Here's how the part is built. I have some questions about the finished solid (model axes, mm). Face numbers are marked on the shaded views. A direction names the side the tool comes from. Give positions to 0.01 mm unless a question says otherwise; leave off trailing zeros. Loops run counter-clockwise (first coordinate to the right, second up) from the corner with the lowest first, then second, coordinate; pieces in that order, holes last. Notation, with made-up numbers: (33.25, 76) -> (55.25, 76) arc R33 ccw to (55.25, 106) -> close; hole circle Ø4 at (-1.5, 32.5). An arc over 180 degrees is marked (long way). Answer in a Markdown table with one row per item. Add a question column.
Item 1: We'd pull the mould along Z, two halves only. Please class the marked faces 1, 2, 3 and 4: released by +Z, released by -Z, zero draft, split by the parting line, or undercut.
Item 2: If I drill on line 1 (Y direction, x = 21, z = 0); line 2 (Y direction, x = -7, z = 0); line 3 (Z direction, x = -8, y = 46), over which ranges is the centre line in solid material (lowest first)?
Item 3: If we section it at C-C (z = 0): Give the number of separate pieces and of enclosed holes in the cut face, then the cut area to 3 significant figures.
Item 4: Which directions (+Z, -Z, +X, -X, +Y, -Y) give clear straight access to the entire face, cutting with the end or side of a thin tool? Please do the marked faces 5, 6 and 7.
Item 5: If we section it at B-B (y = 4): Write out the boundary of the cut face in (x, z), then the cut area to 3 significant figures.
Item 6: For P1, Ø12, axis at x = 18.5, y = 21, coming from the +Z side (1 decimal); P2, Ø6, axis at x = 10, y = 47.5, coming from the +Z side; P3, Ø2.5, axis at x = -8.5, z = 1.5, coming from the -Y side; P4, Ø2, axis at x = 12, y = 8, coming from the -Z side, each with a flat end and sliding along its axis, tell me the tip position at first contact or that it passes through.
Item 7: If we section it at A-A (x = 0): Write out the boundary of the cut face in (y, z).
Item 8: If we section it at D-D (x = 13): Write out the boundary of the cut face in (y, z).
Autodesk Inventor part; units mm, degrees
ref_plane "YZ Plane" through (0, 0, 0) normal (1, 0, 0) x (0, 1, 0)
ref_plane "XZ Plane" through (0, 0, 0) normal (0, 1, 0) x (-1, 0, 0)
ref_plane "XY Plane" through (0, 0, 0) normal (0, 0, 1) x (1, 0, 0)
sketch "Sketch1" plane through (0, 0, 0) normal (0, 1, 0) x (-1, 0, 0)
  circle A0 centre (0, 0) radius 6.15
  line L0 (10, 13) -> (-10, 13)
  line L1 (-10, 13) -> (-10, -13)
  line L2 (-10, -13) -> (10, -13)
  line L3 (10, -13) -> (10, 13)
  dimension "d0" = 12.3
  dimension "d1" = 10
  dimension "d2" = 10
  dimension "d3" = 13
  dimension "d4" = 13
extrude "Extrusion1" add sketch "Sketch1" along normal blind 55
sketch "Sketch2" plane through (10, 0, 13) normal (1, 0, 0) x (0, 0, -1)
  circle A0 centre (13, 4) radius 1.45
  line L0 (0, 0) -> (26, 0)
  circle A1 centre (13, 46) radius 1.45
  line L1 (0, 0) -> (0, 55)
  point P0 (13, 0)
  dimension "d7" = 2.9
  dimension "d8" = 4
  dimension "d9" = 2.9
  dimension "d10" = 46
  dimension "d11" = 13
  dimension "d12" = 13
extrude "Extrusion2" cut sketch "Sketch2" against normal blind 55
sketch "Sketch3" plane through (10, 0, 13) normal (1, 0, 0) x (0, 0, -1)
  circle A0 centre (13, 4) radius 1.45
  circle A1 centre (13, 46) radius 1.45
  line L0 (0, 0) -> (26, 0)
  line L1 (26, 0) -> (26, 55)
  line L2 (0, 55) -> (26, 55)
  line L3 (0, 0) -> (0, 55)
  circle A2 centre (13, 46) radius 5.45
  circle A3 centre (13, 4) radius 5.45
  circle A4 centre (4, 46) radius 1.6
  circle A5 centre (22, 46) radius 1.6
  circle A6 centre (4, 4) radius 1.6
  circle A7 centre (22, 4) radius 1.6
  point P0 (13, 0)
  dimension "d15" = 4
  dimension "d16" = 4
  dimension "d19" = 3.2
  dimension "d20" = 3.2
  dimension "d21" = 3.2
  dimension "d22" = 3.2
  dimension "d23" = 4
  dimension "d24" = 4
  dimension "d25" = 4
  dimension "d26" = 4
extrude "Extrusion3" add sketch "Sketch3" along normal blind 15 contours A3 L0 | L0 A3 | A2
sketch "Sketch6" plane through (-10, 0, 13) normal (0, 0, 1) x (1, 0, 0)
  line L0 (20, 55) -> (0, 55)
  line L1 (20, 0) -> (0, 0)
  line L2 (0, 55) -> (5, 55)
  line L3 (5, 55) -> (5, 0)
  line L4 (5, 0) -> (0, 0)
  line L5 (0, 0) -> (0, 55)
  point P0 (10, 0)
  point P1 (5, 55)
  dimension "d31" = 5
extrude "Extrusion6" add sketch "Sketch6" along normal blind 5
sketch "Sketch7" plane through (10, 0, -13) normal (0, 0, -1) x (-1, 0, 0)
  line L0 (20, 55) -> (20, 0)
  line L1 (20, 0) -> (15, 0)
  line L2 (20, 55) -> (15, 55)
  line L3 (15, 55) -> (15, 0)
  line L4 (15, 0) -> (20, 0)
  line L5 (20, 0) -> (20, 55)
  point P0 (10, 0)
  dimension "d34" = 5
extrude "Extrusion7" add sketch "Sketch7" along normal blind 5
sketch "Sketch8" plane through (0, 0, 0) normal (0, -1, 0) x (1, 0, 0)
  line L0 (10, 13) -> (10, -13)
  line L1 (-10, 18) -> (-10, -18)
  line L2 (10, 13) -> (-10, 13)
  line L3 (-10, 13) -> (-10, 3)
  line L4 (-10, 3) -> (10, 3)
  line L5 (10, 3) -> (10, 13)
  line L6 (10, -13) -> (-5, -13)
  line L7 (10, -13) -> (-10, -13)
  line L8 (-10, -13) -> (-10, -3)
  line L9 (-10, -3) -> (10, -3)
  line L10 (10, -3) -> (10, -13)
  point P0 (0, 0)
  point P1 (10, -3)
  point P2 (-10, -3)
  dimension "d37" = 10
  dimension "d38" = 10
extrude "Extrusion8" add sketch "Sketch8" along normal blind 2 contours L0 L4 L1 L2 | L0 L6 L7 L1 L9
properties part number "Tube_outerhole_template_p1"
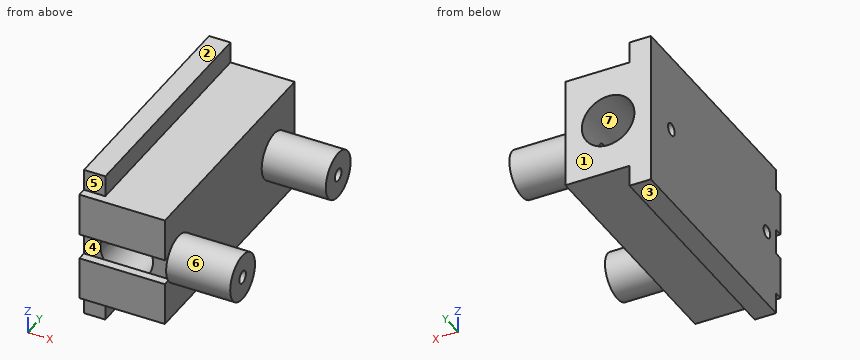
Recorded:
| question | item | result |
|---|---|---|
| 1 | face 1 | zero draft |
| 1 | face 2 | released by +Z |
| 1 | face 3 | released by -Z |
| 1 | face 4 | undercut |
| 2 | line 1 | y = -1.45 to 2.55, 5.45 to 9.45, 40.55 to 44.55, 47.45 to 51.45 |
| 2 | line 2 | y = 0 to 2.55, 5.45 to 44.55, 47.45 to 55 |
| 2 | line 3 | z = -18 to -1.45, 1.45 to 18 |
| 3 | separate pieces | 6 |
| 3 | enclosed holes | 0 |
| 3 | area | 619 mm^2 |
| 4 | face 5 | +Z, +X, -X, -Y |
| 4 | face 6 | +X |
| 4 | face 7 | +Y |
| 5 | outline | (-10, -18) -> (-5, -18) -> (-5, -13) -> (10, -13) -> (10, -5.45) -> (25, -5.45) -> (25, -1.45) -> (5.98, -1.45) arc R6.15 cw to (-5.98, -1.45) -> (-10, -1.45) -> close; (-10, 1.45) -> (-5.98, 1.45) arc R6.15 cw to (5.98, 1.45) -> (25, 1.45) -> (25, 5.45) -> (10, 5.45) -> (10, 13) -> (-5, 13) -> (-5, 18) -> (-10, 18) -> close |
| 5 | area | 549 mm^2 |
| 6 | P1 | passes through |
| 6 | P2 | stops at z = 13 |
| 6 | P3 | stops at y = 0 |
| 6 | P4 | stops at z = -4.55 |
| 7 | outline | (-2, -13) -> (55, -13) -> (55, -6.15) -> (0, -6.15) -> (0, -3) -> (-2, -3) -> close; (-2, 3) -> (0, 3) -> (0, 6.15) -> (55, 6.15) -> (55, 13) -> (-2, 13) -> close |
| 8 | outline | circle Ø10.9 at (4, 0); circle Ø10.9 at (46, 0); hole circle Ø2.9 at (4, 0); hole circle Ø2.9 at (46, 0) |
